Read the model definition and answer for the solid it produces. Units are mm, in the model's axes. A direction names the side the tool comes from. Round coordinates to 2 decimals unless told otherwise and drop trailing zeros. Write each loop counter-clockwise with the first axis right and the second up, starting at its lowest first coordinate (ties: lowest second). Pieces come first, ordered by that corner, then holes. Notation, with made-up numbers: (66, 70) - (89, 70) arc R22 ccw to (89, 108) - close; hole circle Ø10 at (71, 76.25). An arc over 180 degrees is marked (long way). One line per item, written item: value. Start each with the question number.
(1) A cutting plane is placed at A-A, the plane x = 222. Determine the outline of the cut face in (y, z).
(2) Flat-ended cylindrical pins translate along their axes: pin 1 Ø10 at (x, y) = (-17, 19.5) entering from +Z; pin 2 Ø2 at (y, z) = (14, -23.5) entering from -X; pin 3 Ø20 at (x, z) = (111, 3.5) entering from +Y. Find the tip coordinate at first contact, or state that the pin passes through.
(3) The mould has two halves that part along Y. Classify faces 5 (the face through (243, 6, 6)), 6 (the face through (222.317, -2.681, 6.466)), 7 (the face through (198.73, -1.19, 0.26)), 8 (the face through (-4.437, 34.168, -7.587)): +Y half, -Y half, draft (parallel to the pull), parting line (faces both ways), or undercut.
(4) A cutting plane is placed at B-B, the plane x = 118. Determine the outline of the cut face in (y, z).
(5) Find the intervals of material crossed by L1, parallel to Y at x = 229, z = 0; L2, parallel to X at y = -10.5, z = -26; L3, parallel to Y at x = -23, z = -1, in increasing order.
(6) For faces 1 (the face through (122, 26, 9)), 2 (the face through (-33.16, -18.97, 12.1)), 3 (the face through (122.694, -25.296, 16.128)), 4 (the face through (-59, 0, 0)), determine the directions among +Z, -Z, +X, -X, +Y, -Y from which every point of the face is accessible in a straight line to the end or side of a thin tool.
from build123d import *

# Parameters (mm, degrees)
CHAMFER_1_SIZE         = 1
HOLE_WIZARD_M161_D     = 14
HOLE_WIZARD_M161_DEPTH = 40.793975667
HOLE_WIZARD_M161_TIP   = 4.206024333
CUT_EXTRUDE_1_DEPTH    = 7
CUT_EXTRUDE_2_DEPTH    = 5.5


with BuildPart() as part:
    # Эскиз1 → Повернуть1 (revolve)
    with BuildSketch(Plane.XY, mode=Mode.PRIVATE) as revolve_1_sk:
        Polygon((-59, 0), (-59, 22.5), (-9, 22.5), (-9, 35), (0, 35), (0, 30), (243, 30), (243, 0), align=None)
    revolve(revolve_1_sk.sketch.rotate(Axis((-233.488372093, 0, 0), (1, 0, 0)), 90), axis=Axis((-233.488372093, 0, 0), (1, 0, 0)))

    # Фаска1
    chamfer_1_edges = [part.edges().sort_by_distance(p)[0] for p in [
        (243, 0, -30),
        (-59, 0, -22.5),
    ]]
    chamfer(chamfer_1_edges, length=CHAMFER_1_SIZE)

    # Отверстие обработанное метчиком M161
    with Locations(Plane(origin=(243, 0, 0), x_dir=(0, 0, -1), z_dir=(1, 0, 0))):
        with Locations((0, 0)):
            Hole(HOLE_WIZARD_M161_D / 2, depth=HOLE_WIZARD_M161_DEPTH)
            with Locations((0, 0, -(HOLE_WIZARD_M161_DEPTH + HOLE_WIZARD_M161_TIP / 2))):  # 118° drill point
                Cone(0, HOLE_WIZARD_M161_D / 2, HOLE_WIZARD_M161_TIP, mode=Mode.SUBTRACT)

    # Эскиз4 → Вырез-Вытянуть1 (cut)
    with BuildSketch(Plane(origin=(0, 30, 0), x_dir=(1, 0, 0), z_dir=(0, 1, 0))):
        with BuildLine():
            Line((167, -9), (75, -9))
            ThreePointArc((75, -9), (66, 0), (75, 9))
            Line((75, 9), (167, 9))
            ThreePointArc((167, 9), (176, 0), (167, -9))
        make_face()
    extrude(amount=-CUT_EXTRUDE_1_DEPTH, mode=Mode.SUBTRACT)

    # Эскиз5 → Вырез-Вытянуть2 (cut)
    with BuildSketch(Plane(origin=(0, 22.5, 0), x_dir=(1, 0, 0), z_dir=(0, 1, 0))):
        with BuildLine():
            Line((-47, 7), (-21, 7))
            ThreePointArc((-21, 7), (-14, 0), (-21, -7))
            Line((-21, -7), (-47, -7))
            ThreePointArc((-47, -7), (-54, 0), (-47, 7))
        make_face()
    extrude(amount=-CUT_EXTRUDE_2_DEPTH, mode=Mode.SUBTRACT)


solid = part.part
Here are the results:
1. outline: circle Ø60 at (0, 0); hole circle Ø14 at (0, 0)
2. pin 1: z = 17.2
2. pin 2: x = -9
2. pin 3: y = 28.62
3. face 5: draft
3. face 6: undercut
3. face 7: undercut
3. face 8: parting line
4. outline: (23, -9) - (23, 9) - (28.62, 9) arc R30 ccw (long way) to (28.62, -9) - close
5. L1: -30 to -7, 7 to 30
5. L2: -9 to 243
5. L3: -22.48 to 17
6. face 1: +Y
6. face 2: -X
6. face 3: +X
6. face 4: +Z, -Z, -X, +Y, -Y
